CAD build for the part. Positions are in the model's coordinates, mm. Face numbers are marked on the shaded views. A direction names the side the tool comes from. Coordinates: 2 decimals unless noted, no trailing zeros. Loops run counter-clockwise (first coordinate to the right, second up) from the corner with the lowest first, then second, coordinate; pieces in that order, holes last. Notation, with made-up numbers: (60, 48) -> (118, 48) arc R18 ccw to (118, 71) -> close; hole circle Ø1 at (59.25, 43.5). An arc over 180 degrees is marked (long way). Return JSON: item names as keys, results as strings. Group by question number.
(1) Saw through at D-D on x = -9.25. Write the cut outline in (y, z).
(2) Mould opens along Z. For the marked faces 1 and 2 say: pulls with the +Z half, pulls with the -Z half, needs draft (parallel to the pull), parting line crosses it, or undercut.
(3) Saw through at B-B on y = 20. Write the cut outline in (x, z), then the cut area to 3 significant figures.
(4) Saw through at C-C on x = -3.5. Write the cut outline in (y, z), then the cut area to 3 significant figures.
(5) Saw through at A-A on y = 34. Write the cut outline in (x, z).
(6) Tool access for the marked faces 3, 4 and 5: list every direction of +Z, -Z, +X, -X, +Y, -Y with a clear straight run to the whole face (end or side of a thin tool).
(7) Probe L1, parallel to Z at x = -9, y = 33.5 (3 decimals); L2, parallel to Z at x = -7, y = 17.5; L3, parallel to Z at x = -12, y = 6. List the from-to ranges inside material, lowest first.
(8) Flat gauge pins, fed straight in: pin 1 Ø5.5 at (y, z) = (34, 16.79) entering from -X; pin 2 Ø4.5 at (y, z) = (6, 16.79) entering from +X; pin 3 Ø1 at (x, y) = (-11.5, 28.5) entering from +Z; pin 4 Ø4.5 at (y, z) = (6, -27.77) entering from +X. Where does each tip first touch, or does it go through?
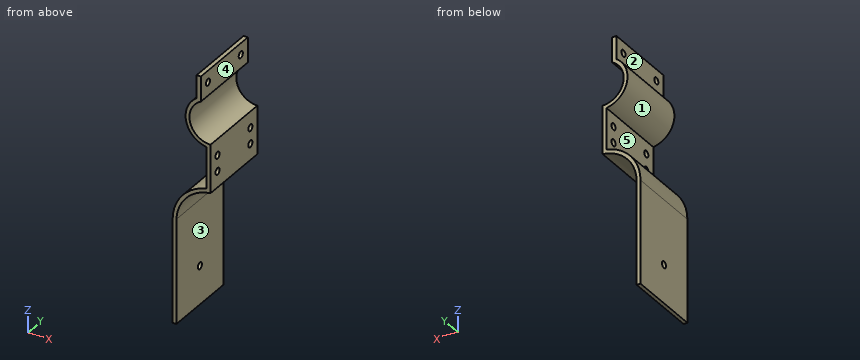
```python
from build123d import *

# Parameters (mm, degrees)
BOSS_EXTRUDE1_DEPTH     = 40
CUT_EXTRUDE1_DEPTH      = 118.727312348
CUT_EXTRUDE1_DEPTH_BACK = 118.727312348
SKETCH3_R               = 1.75


with BuildPart() as part:
    # Sketch1 → Boss-Extrude1 (new body)
    with BuildSketch(Plane(origin=(0, 0, 0), x_dir=(1, 0, 0), z_dir=(0, 1, 0))):
        with BuildLine():
            Line((0, 11), (0, 36.098802305))
            ThreePointArc((0, 36.098802305), (-12.451450114, 42.224601119), (-17.776180484, 55.03909555))
            Line((-17.776180484, 55.03909555), (-17.776180484, 109.287361941))
            Line((-17.776180484, 109.287361941), (-19.776180484, 109.287361941))
            Line((-19.776180484, 109.287361941), (-19.776180484, 55.700978031))
            ThreePointArc((-19.776180484, 55.700978031), (-14.749868805, 41.814960106), (-2, 34.363373136))
            Line((-2, 34.363373136), (-2, 12.845232579))
            ThreePointArc((-2, 12.845232579), (-12.692786177, 2.809480212), (-7.234039362, -10.801327442))
            Line((-7.234039362, -10.801327442), (-7.234039362, -22.783960598))
            Line((-7.234039362, -22.783960598), (-5, -22.783960598))
            Line((-5, -22.783960598), (-5, -9.797958971))
            ThreePointArc((-5, -9.797958971), (-10.695268783, 2.571230378), (0, 11))
        make_face()
    extrude(amount=BOSS_EXTRUDE1_DEPTH)

    # Sketch3 → Cut-Extrude1 (cut, two sides: drawn at the far end of the back side and taken through both)
    with BuildSketch(Plane.ZY.offset(2).offset(-CUT_EXTRUDE1_DEPTH_BACK)):
        with Locations((-27.77399295, 34)):
            Circle(SKETCH3_R)
        with Locations((-19.434612764, 34)):
            Circle(SKETCH3_R)
        with Locations((16.79264402, 34)):
            Circle(SKETCH3_R)
        with Locations((-89.287361941, 20)):
            Circle(SKETCH3_R)
        with Locations((16.79264402, 6)):
            Circle(SKETCH3_R)
        with Locations(Location((-19.434612764, 6, 0), (0, 0, 180))):
            Circle(SKETCH3_R)
        with Locations(Location((-27.77399295, 6, 0), (0, 0, 180))):
            Circle(SKETCH3_R)
    extrude(amount=CUT_EXTRUDE1_DEPTH + CUT_EXTRUDE1_DEPTH_BACK, mode=Mode.SUBTRACT)


solid = part.part
```
Geometry results:
{
 "1": {"outline": "(0, -39.47) -> (40, -39.47) -> (40, -37.1) -> (0, -37.1) -> close; (0, -9.13) -> (40, -9.13) -> (40, -5.95) -> (0, -5.95) -> close; (0, 5.95) -> (40, 5.95) -> (40, 9.13) -> (0, 9.13) -> close"},
 "2": {"face 1": "undercut", "face 2": "needs draft"},
 "3": {"outline": "(-19.78, -109.29) -> (-17.78, -109.29) -> (-17.78, -91.04) -> (-19.78, -91.04) -> close; (-19.78, -87.54) -> (-17.78, -87.54) -> (-17.78, -55.04) arc R19.7 cw to (0, -36.1) -> (0, -11) arc R11 cw to (-5, 9.8) -> (-5, 22.78) -> (-7.23, 22.78) -> (-7.23, 10.8) arc R13 ccw to (-2, -12.85) -> (-2, -34.36) arc R21.69 ccw to (-19.78, -55.7) -> close", "area": "294 mm²"},
 "4": {"outline": "(0, -36.76) -> (40, -36.76) -> (40, -34.69) -> (0, -34.69) -> close; (0, -12.52) -> (40, -12.52) -> (40, -10.43) -> (0, -10.43) -> close", "area": "166 mm²"},
 "5": {"outline": "(-19.78, -109.29) -> (-17.78, -109.29) -> (-17.78, -55.04) arc R19.7 cw to (0, -36.1) -> (0, -29.52) -> (-2, -29.52) -> (-2, -34.36) arc R21.69 ccw to (-19.78, -55.7) -> close; (-7.23, 10.8) arc R13 ccw to (-2, -12.85) -> (-2, -17.68) -> (0, -17.68) -> (0, -11) arc R11 cw to (-5, 9.8) -> (-5, 15.04) -> (-7.23, 15.04) -> close; (-7.23, 18.54) -> (-5, 18.54) -> (-5, 22.78) -> (-7.23, 22.78) -> close; (-2, -26.02) -> (0, -26.02) -> (0, -21.18) -> (-2, -21.18) -> close"},
 "6": {"face 3": "-Z, +X, +Y, -Y", "face 4": "+Z, +X, +Y, -Y", "face 5": "-X, +Y, -Y"},
 "7": {"L1": "-39.305 to -36.954, -9.381 to -6.325, 6.325 to 9.381", "L2": "-38.14 to -35.92, -10.95 to -8.49, 8.49 to 22.78", "L3": "-41.76 to -39.06, -5 to 5"},
 "8": {"pin 1": "x = -7.23", "pin 2": "x = -5", "pin 3": "z = 6.93", "pin 4": "x = 0"}
}
